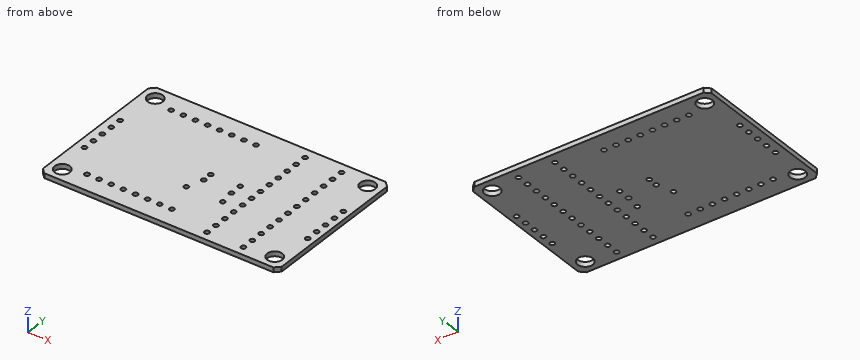
from build123d import *

# Parameters (mm, degrees)
SKETCH1_W           = 50
SKETCH1_H           = 32
SKETCH1_R           = 1.6
BOSS_EXTRUDE1_DEPTH = 1
SKETCH3_R           = 0.5
CUT_EXTRUDE1_DEPTH  = 1
CHAMFER1_SIZE       = 1


with BuildPart() as part:
    # Sketch1 → Boss-Extrude1 (new body)
    with BuildSketch(Plane.XY):
        Rectangle(SKETCH1_W, SKETCH1_H)
        with Locations((-22.25, -13.25)):
            Circle(SKETCH1_R, mode=Mode.SUBTRACT)
        with Locations((22.25, -13.25)):
            Circle(SKETCH1_R, mode=Mode.SUBTRACT)
        with Locations((22.25, 13.25)):
            Circle(SKETCH1_R, mode=Mode.SUBTRACT)
        with Locations((-22.25, 13.25)):
            Circle(SKETCH1_R, mode=Mode.SUBTRACT)
    extrude(amount=BOSS_EXTRUDE1_DEPTH)

    # Sketch3 → Cut-Extrude1 (cut)
    with BuildSketch(Plane(origin=(0, 0, 0), x_dir=(-1, 0, 0), z_dir=(0, 0, -1))):
        with Locations((-23.5, 4.6)):
            Circle(SKETCH3_R)
        with Locations((-23.5, 2.06)):
            Circle(SKETCH3_R)
        with Locations((-23.5, -0.48)):
            Circle(SKETCH3_R)
        with Locations((-23.5, -3.02)):
            Circle(SKETCH3_R)
        with Locations((-23.5, -5.56)):
            Circle(SKETCH3_R)
        with Locations((-16.3, 13.85)):
            Circle(SKETCH3_R)
        with Locations((-16.3, 11.31)):
            Circle(SKETCH3_R)
        with Locations((-16.3, 8.77)):
            Circle(SKETCH3_R)
        with Locations((-16.3, 6.23)):
            Circle(SKETCH3_R)
        with Locations((-16.3, 3.69)):
            Circle(SKETCH3_R)
        with Locations((-16.3, 1.15)):
            Circle(SKETCH3_R)
        with Locations((-16.3, -1.39)):
            Circle(SKETCH3_R)
        with Locations((-16.3, -3.93)):
            Circle(SKETCH3_R)
        with Locations((-16.3, -6.47)):
            Circle(SKETCH3_R)
        with Locations((-16.3, -9.01)):
            Circle(SKETCH3_R)
        with Locations((-16.3, -11.55)):
            Circle(SKETCH3_R)
        with Locations((-16.3, -14.09)):
            Circle(SKETCH3_R)
        with Locations((-8.68, 13.85)):
            Circle(SKETCH3_R)
        with Locations((-8.68, 11.31)):
            Circle(SKETCH3_R)
        with Locations((-8.68, 8.77)):
            Circle(SKETCH3_R)
        with Locations((-8.68, 6.23)):
            Circle(SKETCH3_R)
        with Locations((-8.68, 3.69)):
            Circle(SKETCH3_R)
        with Locations((-8.68, 1.15)):
            Circle(SKETCH3_R)
        with Locations((-8.68, -1.39)):
            Circle(SKETCH3_R)
        with Locations((-8.68, -3.93)):
            Circle(SKETCH3_R)
        with Locations((-8.68, -6.47)):
            Circle(SKETCH3_R)
        with Locations((-8.68, -9.01)):
            Circle(SKETCH3_R)
        with Locations((-8.68, -11.55)):
            Circle(SKETCH3_R)
        with Locations((-8.68, -14.09)):
            Circle(SKETCH3_R)
        with Locations((18, 12)):
            Circle(SKETCH3_R)
        with Locations((15.46, 12)):
            Circle(SKETCH3_R)
        with Locations((12.92, 12)):
            Circle(SKETCH3_R)
        with Locations((10.38, 12)):
            Circle(SKETCH3_R)
        with Locations((7.84, 12)):
            Circle(SKETCH3_R)
        with Locations((5.3, 12)):
            Circle(SKETCH3_R)
        with Locations((2.76, 12)):
            Circle(SKETCH3_R)
        with Locations((0.22, 12)):
            Circle(SKETCH3_R)
        with Locations((18, -12)):
            Circle(SKETCH3_R)
        with Locations((15.46, -12)):
            Circle(SKETCH3_R)
        with Locations((12.92, -12)):
            Circle(SKETCH3_R)
        with Locations((10.38, -12)):
            Circle(SKETCH3_R)
        with Locations((7.84, -12)):
            Circle(SKETCH3_R)
        with Locations((5.3, -12)):
            Circle(SKETCH3_R)
        with Locations((2.76, -12)):
            Circle(SKETCH3_R)
        with Locations((0.22, -12)):
            Circle(SKETCH3_R)
        with Locations((23.1, 4.4)):
            Circle(SKETCH3_R)
        with Locations((23.1, 1.86)):
            Circle(SKETCH3_R)
        with Locations((23.1, -0.68)):
            Circle(SKETCH3_R)
        with Locations((23.1, -3.22)):
            Circle(SKETCH3_R)
        with Locations((23.1, -5.76)):
            Circle(SKETCH3_R)
        with Locations((-5, 0.4)):
            Circle(SKETCH3_R)
        with Locations((-5, -2.14)):
            Circle(SKETCH3_R)
        with Locations((-5.37, -5.1)):
            Circle(SKETCH3_R)
        with Locations((2.25, -5.1)):
            Circle(SKETCH3_R)
        with Locations((1.1, 0.3)):
            Circle(SKETCH3_R)
        with Locations((1.1, -1.7)):
            Circle(SKETCH3_R)
    extrude(amount=-CUT_EXTRUDE1_DEPTH, mode=Mode.SUBTRACT)

    # Chamfer1
    chamfer1_edges = [part.edges().sort_by_distance(p)[0] for p in [
        (-25, 16, 0.5),
        (25, 16, 0.5),
        (25, -16, 0.5),
        (-25, -16, 0.5),
    ]]
    chamfer(chamfer1_edges, length=CHAMFER1_SIZE)


solid = part.part
Check sheet for the modelled part. Datum: model origin and axes. Units: mm. Give positions to 0.01 mm unless a question says otherwise; leave off trailing zeros. Order: outer loops, then holes, each group sorted by start corner. A loop starts at its lowest first (then second) coordinate and runs counter-clockwise, first axis right, second up. Notation, with made-up numbers: M -31.5,77 L 18.5,77 A18 cw 18.5,88 Z; hole C 86.25,-8.5 d2. An arc over 180 degrees is marked long. Answer as CSV lines item,"result". Start each with the question number.
Item 1: Gauge pin test, flat end, axial feed: P1, Ø1.9, axis at x = -22.25, y = 13.25, coming from the +Z side. Record the tip position at first contact, or that the pin passes through.
Item 2: Cross-section at C-C on z = 0.45. State how many separate pieces and enclosed holes the cut face has, plus the area to 3 significant figures.
Item 3: Thickness scan on line 1 (Y direction, x = -10.38, z = 0.5); line 2 (Y direction, x = 5, z = 0.95); line 3 (X direction, y = 0.5, z = 0.35). Record the ranges inside material, lowest first. Write a range as [from, to].
Item 4: Cross-section at B-B on y = 13.85. Enter the section's corners in (x, z), plus the area to 3 significant figures.
Item 5: Cross-section at A-A on x = -18. Enter the section's corners in (y, z), plus the area to 3 significant figures.
Established:
1,P1,"passes through"
2,separate pieces,"1"
2,enclosed holes,"60"
2,area,"1,520 mm^2"
3,line 1,"y = [-16, -12.5], [-11.5, 11.5], [12.5, 16]"
3,line 2,"y = [-16, -5.44], [-4.76, -2.64], [-1.64, -0.1], [0.9, 16]"
3,line 3,"x = [-25, -1.56], [-0.64, 4.51], [5.49, 25]"
4,outline,"M -25,0 L -23.73,0 L -23.73,1 L -25,1 Z; M -20.77,0 L 8.18,0 L 8.18,1 L -20.77,1 Z; M 9.18,0 L 15.8,0 L 15.8,1 L 9.18,1 Z; M 16.8,0 L 20.77,0 L 20.77,1 L 16.8,1 Z; M 23.73,0 L 25,0 L 25,1 L 23.73,1 Z"
4,area,"42.1 mm^2"
5,outline,"M -16,0 L -12.5,0 L -12.5,1 L -16,1 Z; M -11.5,0 L 11.5,0 L 11.5,1 L -11.5,1 Z; M 12.5,0 L 16,0 L 16,1 L 12.5,1 Z"
5,area,"30.0 mm^2"
